from build123d import *

# Parameters (mm, degrees)
SKETCH1_R           = 3.2639
BOSS_EXTRUDE1_DEPTH = 1.5875


with BuildPart() as part:
    # Sketch1 → Boss-Extrude1 (new, symmetric)
    with BuildSketch(Plane(origin=(0, 0, 0), x_dir=(0, 0, -1), z_dir=(1, 0, 0))):
        with BuildLine():
            Line((-38.1, 9.525), (-38.1, -9.525))
            Line((-38.1, -9.525), (0.516366314, -6.418161656))
            ThreePointArc((0.516366314, -6.418161656), (6.4389, 0), (0.516366314, 6.418161656))
            Line((0.516366314, 6.418161656), (-38.1, 9.525))
        make_face()
        Circle(SKETCH1_R, mode=Mode.SUBTRACT)
    extrude(amount=BOSS_EXTRUDE1_DEPTH, both=True)


solid = part.part
Source: CAD feature listing. Evaluate the final solid. Frame: model axes, mm. Round coordinates to 2 decimals unless told otherwise and drop trailing zeros. Order: outer loops, then holes, each group sorted by start corner. A loop starts at its lowest first (then second) coordinate and runs counter-clockwise, first axis right, second up. Notation, with made-up numbers: (38.5, -0.5) - (57.5, -0.5) arc R29 ccw to (57.5, 25.5) - close; hole circle Ø3 at (-1.75, 75.25). An arc over 180 degrees is marked (long way). Use a Markdown table: item, result. Add a question column.
1. Section query A-A (y = 0). Return the cut outline in (x, z), then the cut area to 3 significant figures.
2. Section query B-B (z = 0). Return the cut outline in (x, y), then the cut area to 3 significant figures.
3. Line query: probe 1 along Z at (x, y) = (0.85, -3); probe 2 along Z at (x, y) = (-1.3, -0.25); probe 3 along Y at (x, z) = (-0.8, 0). Output: solid intervals per line, ascending.
4. Section query C-C (x = 0.5). Return the cut outline in (y, z) (3 decimals).
5. Section query D-D (z = 10.5). Return the cut outline in (x, y), then the cut area to 3 significant figures.
6. Mould query, pull axis Z, two halves, no side actions, for faces 1 (the flat face through (0, 0, 38.1)), 2 (the cylindrical face through (-0.022, -3.186, 0.708)), 3 (the flat face through (0.022, -7.993, 19.062)), 4 (the flat face through (-1.588, 0, 21)). Classes: +Z half, -Z half, draft (parallel to the pull), parting line (faces both ways), or undercut.
Derived:
| question | item | result |
|---|---|---|
| 1 | outline | (-1.59, -6.44) - (1.59, -6.44) - (1.59, -3.26) - (-1.59, -3.26) - close; (-1.59, 3.26) - (1.59, 3.26) - (1.59, 38.1) - (-1.59, 38.1) - close |
| 1 | area | 121 mm2 |
| 2 | outline | (-1.59, -6.46) - (1.59, -6.46) - (1.59, -3.26) - (-1.59, -3.26) - close; (-1.59, 3.26) - (1.59, 3.26) - (1.59, 6.46) - (-1.59, 6.46) - close |
| 2 | area | 20.3 mm2 |
| 3 | probe 1 | -5.7 to -1.29, 1.29 to 38.1 |
| 3 | probe 2 | -6.43 to -3.25, 3.25 to 38.1 |
| 3 | probe 3 | -6.46 to -3.26, 3.26 to 6.46 |
| 4 | outline | (-9.525, 38.1) - (-6.418, -0.516) arc R6.439 ccw to (6.418, -0.516) - (9.525, 38.1) - close; hole circle Ø6.528 at (0, 0) |
| 5 | outline | (-1.59, -7.3) - (1.59, -7.3) - (1.59, 7.3) - (-1.59, 7.3) - close |
| 5 | area | 46.4 mm2 |
| 6 | face 1 | +Z half |
| 6 | face 2 | undercut |
| 6 | face 3 | -Z half |
| 6 | face 4 | draft |
